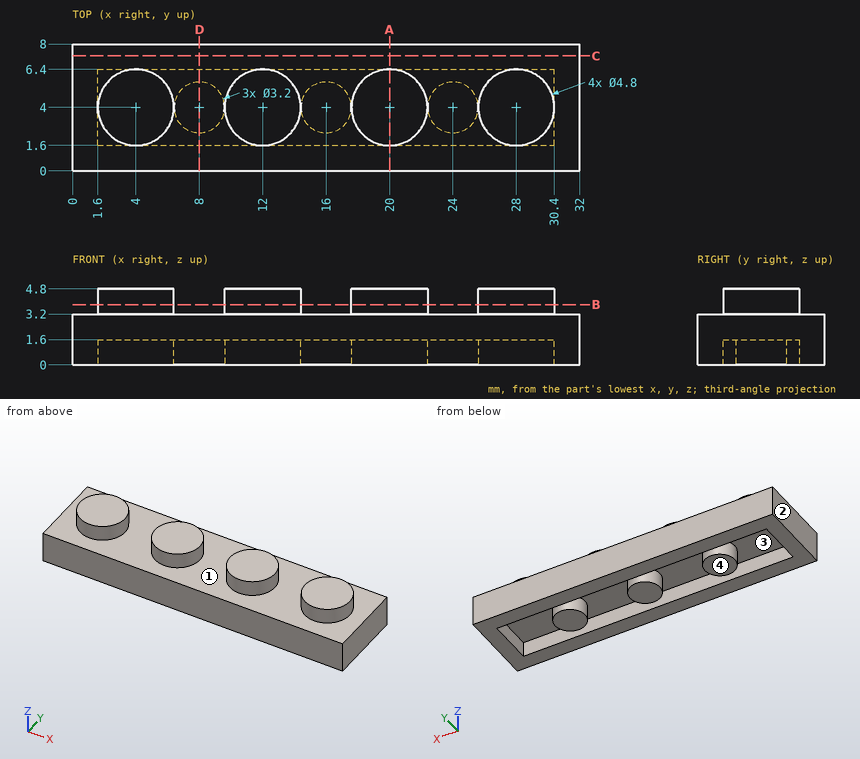
The figure shows three views and two pictorial views of one solid part (mm, origin at its lowest corner). Answer the questions. Round coordinates to 2 decimals unless told otherwise and drop trailing zeros. Write each loop counter-clockwise with the first axis right and the second up, starting at its lowest first coordinate (ties: lowest second). Pieces come first, ordered by that corner, then holes. Notation, with made-up numbers: M 28.25,62 L 43.25,62 A22 ccw 43.25,83 Z; hole C 30.25,18.25 d5. An arc over 180 degrees is marked long. Use a Markdown table: item, result.
1) Flat-ended cylindrical pins translate along their axes: pin 1 (0.8 mm diameter, centred on y = 3, z = 1, fed in from -X); pin 2 (2.5 mm diameter, centred on x = 13, y = 3, fed in from -Z); pin 3 (1 mm diameter, centred on x = 8, z = 4, fed in from +Y) (3 decimals). Find the tip coordinate at first contact, or state that the pin passes through.
Taken from the geometry:
| item | result |
|---|---|
| pin 1 | stops at x = 0 |
| pin 2 | stops at z = 1.6 |
| pin 3 | passes through |
2) The part is cut by section A-A on x = 20. Give the vertices of the cut face in (y, z).
Taken from the geometry:
| item | result |
|---|---|
| outline | M 0,0 L 1.6,0 L 1.6,1.6 L 6.4,1.6 L 6.4,0 L 8,0 L 8,3.2 L 6.4,3.2 L 6.4,4.8 L 1.6,4.8 L 1.6,3.2 L 0,3.2 Z |
3) The part is cut by section B-B on z = 3.8. Give the vertices of the cut face in (x, y).
Taken from the geometry:
| item | result |
|---|---|
| outline | C 4,4 d4.8; C 12,4 d4.8; C 20,4 d4.8; C 28,4 d4.8 |
4) Determine the mould class of the marked faces 1, 2, 3 and 4 for opening direction X: pulls with the +X half, pulls with the -X half, needs draft (parallel to the pull), parting line crosses it, or undercut.
Taken from the geometry:
| item | result |
|---|---|
| face 1 | undercut |
| face 2 | pulls with the -X half |
| face 3 | undercut |
| face 4 | needs draft |
5) The part is cut by section D-D on x = 8. Give the vertices of the cut face in (y, z).
Taken from the geometry:
| item | result |
|---|---|
| outline | M 0,0 L 1.6,0 L 1.6,1.6 L 2.4,1.6 L 2.4,0 L 5.6,0 L 5.6,1.6 L 6.4,1.6 L 6.4,0 L 8,0 L 8,3.2 L 0,3.2 Z |
6) The part is cut by section C-C on y = 7.25. Give the vertices of the cut face in (x, z), plus the area to 3 significant figures.
Taken from the geometry:
| item | result |
|---|---|
| outline | M 0,0 L 32,0 L 32,3.2 L 0,3.2 Z |
| area | 102 mm2 |
7) Consider line 1 (Y direction, x = 10.5, z = 0.8); line 2 (Z direction, x = 8.5, y = 4.5); line 3 (X direction, y = 3.25, z = 3.9). Determine where each line is inside the solid, lowest interval first. Write a range as [from, to].
Taken from the geometry:
| item | result |
|---|---|
| line 1 | y = [0, 1.6], [6.4, 8] |
| line 2 | z = [0, 3.2] |
| line 3 | x = [1.72, 6.28], [9.72, 14.28], [17.72, 22.28], [25.72, 30.28] |
